Geometry check sheet. Reference: the model listing, model coordinates, mm. A direction names the side the tool comes from. Coordinates: 2 decimals unless noted, no trailing zeros. Write each loop counter-clockwise with the first axis right and the second up, starting at its lowest first coordinate (ties: lowest second). Pieces come first, ordered by that corner, then holes. Notation, with made-up numbers: M -34.5,60.5 L -21.5,60.5 A37 ccw -21.5,98.5 Z; hole C 79,-21 d9. An arc over 180 degrees is marked long. Write item = value, one per line. Start each with the question number.
```python
from build123d import *

# Parameters (mm, degrees)
SKETCH1_R           = 1.5
BOSS_EXTRUDE1_DEPTH = 1
SKETCH2_W           = 15.22
SKETCH2_H           = 11.45
BOSS_EXTRUDE2_DEPTH = 5.3
SKETCH3_W           = 13.43
SKETCH3_H           = 1.95
BOSS_EXTRUDE3_DEPTH = 3.5
SKETCH5_W           = 7.6
SKETCH5_H           = 3.8
BOSS_EXTRUDE4_DEPTH = 1.65
SKETCH4_W           = 13.22
SKETCH4_H           = 3.3
SKETCH4_W_2         = 5.6
SKETCH4_H_2         = 1.65
SKETCH4_W_3         = 1.3
SKETCH4_H_3         = 1
CUT_EXTRUDE1_DEPTH  = 9.3
SKETCH6_W           = 0.8
SKETCH6_H           = 0.8
BOSS_EXTRUDE5_DEPTH = 5.95
SKETCH7_W           = 4
SKETCH7_H           = 5.1
BOSS_EXTRUDE6_DEPTH = 1.6
FILLET1_R           = 0.25


with BuildPart() as part:
    # Sketch1 → Boss-Extrude1 (new body)
    with BuildSketch(Plane(origin=(0, 0, 0), x_dir=(1, 0, 0), z_dir=(0, 1, 0))):
        with BuildLine():
            ThreePointArc((-11.9, -8.825), (-10.999353352, -10.999353352), (-8.825, -11.9))
            Line((-8.825, -11.9), (8.825, -11.9))
            ThreePointArc((8.825, -11.9), (10.999353352, -10.999353352), (11.9, -8.825))
            Line((11.9, -8.825), (11.9, 8.825))
            ThreePointArc((11.9, 8.825), (10.999353357, 10.999353347), (8.825000015, 11.9))
            Line((8.825000015, 11.9), (-8.825, 11.9))
            ThreePointArc((-8.825, 11.9), (-10.999353347, 10.999353357), (-11.9, 8.825000015))
            Line((-11.9, 8.825000015), (-11.9, -8.825))
        make_face()
        with Locations((8.825, -8.825)):
            Circle(SKETCH1_R, mode=Mode.SUBTRACT)
        with Locations((-8.825, -8.825)):
            Circle(SKETCH1_R, mode=Mode.SUBTRACT)
        with Locations((-8.825, 8.825)):
            Circle(SKETCH1_R, mode=Mode.SUBTRACT)
        with Locations((8.825, 8.825)):
            Circle(SKETCH1_R, mode=Mode.SUBTRACT)
    extrude(amount=BOSS_EXTRUDE1_DEPTH)

    # Sketch2 → Boss-Extrude2 (add)
    with BuildSketch(Plane(origin=(0, 1, 0), x_dir=(1, 0, 0), z_dir=(0, 1, 0))):
        Rectangle(SKETCH2_W, SKETCH2_H)
    extrude(amount=BOSS_EXTRUDE2_DEPTH)

    # Sketch3 → Boss-Extrude3 (add)
    with BuildSketch(Plane(origin=(0, 1, 0), x_dir=(1, 0, 0), z_dir=(0, 1, 0))):
        with Locations((0, 6.7)):
            Rectangle(SKETCH3_W, SKETCH3_H)
    extrude(amount=BOSS_EXTRUDE3_DEPTH)

    # Sketch5 → Boss-Extrude4 (add)
    with BuildSketch(Plane(origin=(0, 6.3, 0), x_dir=(1, 0, 0), z_dir=(0, 1, 0))):
        with Locations((0, -3.825)):
            Rectangle(SKETCH5_W, SKETCH5_H)
    extrude(amount=BOSS_EXTRUDE4_DEPTH)

    # Sketch4 → Cut-Extrude1 (cut)
    with BuildSketch(Plane.XY.offset(5.725)):
        with Locations((0, 3.65)):
            Rectangle(SKETCH4_W, SKETCH4_H)
        with Locations((0, 6.125)):
            Rectangle(SKETCH4_W_2, SKETCH4_H_2)
        with Locations((-3.76, 1.5)):
            Rectangle(SKETCH4_W_3, SKETCH4_H_3)
        with Locations((3.76, 1.5)):
            Rectangle(SKETCH4_W_3, SKETCH4_H_3)
    extrude(amount=-CUT_EXTRUDE1_DEPTH, mode=Mode.SUBTRACT)

    # Sketch6 → Boss-Extrude5 (add)
    with BuildSketch(Plane.XY.offset(-3.575)):
        with Locations((2.54, 3.65)):
            Rectangle(SKETCH6_W, SKETCH6_H)
        with Locations((0, 3.65)):
            Rectangle(SKETCH6_W, SKETCH6_H)
        with Locations((5.08, 3.65)):
            Rectangle(SKETCH6_W, SKETCH6_H)
        with Locations((-2.54, 3.65)):
            Rectangle(SKETCH6_W, SKETCH6_H)
        with Locations((-5.08, 3.65)):
            Rectangle(SKETCH6_W, SKETCH6_H)
    extrude(amount=BOSS_EXTRUDE5_DEPTH)

    # Sketch7 → Boss-Extrude6 (add)
    with BuildSketch(Plane.XZ):
        Rectangle(SKETCH7_W, SKETCH7_H)
    extrude(amount=BOSS_EXTRUDE6_DEPTH)

    # Fillet1
    fillet1_edges = [part.edges().sort_by_distance(p)[0] for p in [
        (2, -1.6, 0),
        (0, -1.6, 2.55),
        (-2, -1.6, 0),
        (0, -1.6, -2.55),
    ]]
    fillet(fillet1_edges, radius=FILLET1_R)


solid = part.part
```
Q1. Gauge pin test, flat ends, axial feed: pin 1 (1 mm diameter, centred on y = 6.5, z = 6, fed in from +X); pin 2 (1.5 mm diameter, centred on y = 6.5, z = 8, fed in from +X) (3 decimals); pin 3 (2 mm diameter, centred on x = 6, y = 4.5, fed in from +Z) (3 decimals); pin 4 (1.6 mm diameter, centred on x = 2.5, y = 5, fed in from -Z) (3 decimals). Record the tip position at first contact, or that the pin passes through.
Q2. Draft check along X on faces 6 (the face through (0, 7.95, 4)), 7 (the face through (-3.8, 7, 4)), 8 (the face through (4.41, 1.5, 1.1)), 9 (the face through (7.61, 4, 0)). Enter one of: pulls with the +X half, pulls with the -X half, needs draft (parallel to the pull), parting line crosses it, or undercut.
Q3. Set-up check for faces 1 (the face through (-7.61, 4, 0)), 2 (the face through (0, 7.3, 5.725)), 3 (the face through (11.9, 0.5, 0.1)), 4 (the face through (7.635, 0.493, 9.738)), 5 (the face through (-5, 4.05, -1)): record each of +Z, -Z, +X, -X, +Y, -Y from which the full face is reachable in a straight line by a thin tool's end or side.
Q4. Cross-section at D-D on x = 6. Enter the section's corners in (y, z) (3 decimals).
Q5. Cross-section at B-B on y = 2.5. Enter the section's corners in (x, z) (3 decimals).
Q6. Cross-section at A-A on x = 1.25. Enter the section's corners in (y, z) (3 decimals).
Q7. Scan lines: L1, parallel to X at y = 1.25, z = 4.25; L2, parallel to Y at x = -4.25, z = -3.5; L3, parallel to X at y = 5.5, z = 1.75. Record each from-to range of solid material in increasing order.
Q8. Cross-section at C-C on z = 9.75. Enter the section's corners in (x, y), and give its area (3 significant figures).
Values found:
q1.pin_1 = 7.61
q1.pin_2 = through
q1.pin_3 = 5.725
q1.pin_4 = -7.675
q2.face_6 = needs draft
q2.face_7 = pulls with the -X half
q2.face_8 = undercut
q2.face_9 = pulls with the +X half
q3.face_1 = +Z, -Z, -X, +Y
q3.face_2 = +Z, +X, -X, +Y
q3.face_3 = +Z, -Z, +X, +Y, -Y
q3.face_4 = +Y, -Y
q3.face_5 = +Z
q4.outline = M 0,-11.9 L 1,-11.9 L 1,-7.675 L 4.5,-7.675 L 4.5,-5.725 L 6.3,-5.725 L 6.3,5.725 L 5.3,5.725 L 5.3,-3.575 L 2,-3.575 L 2,5.725 L 1,5.725 L 1,11.9 L 0,11.9 Z
q5.outline = M -7.61,-5.725 L -6.715,-5.725 L -6.715,-7.675 L 6.715,-7.675 L 6.715,-5.725 L 7.61,-5.725 L 7.61,5.725 L 6.61,5.725 L 6.61,-3.575 L -6.61,-3.575 L -6.61,5.725 L -7.61,5.725 Z
q6.outline = M -1.6,-2.3 A0.25 ccw -1.35,-2.55 L 0,-2.55 L 0,-11.9 L 1,-11.9 L 1,-7.675 L 4.5,-7.675 L 4.5,-5.725 L 6.3,-5.725 L 6.3,-3.575 L 2,-3.575 L 2,5.725 L 1,5.725 L 1,11.9 L 0,11.9 L 0,2.55 L -1.35,2.55 A0.25 ccw -1.6,2.3 Z; M 6.95,1.925 L 7.95,1.925 L 7.95,5.725 L 6.95,5.725 Z
q7.L1 = -7.61 to -4.41, -3.11 to 3.11, 4.41 to 7.61
q7.L2 = 0 to 1, 5.3 to 6.3
q7.L3 = -7.61 to -2.8, 2.8 to 7.61
q8.outline = M -11.76,0 L -10.01,0 L -10.01,1 L -11.76,1 Z; M -7.64,0 L 7.64,0 L 7.64,1 L -7.64,1 Z; M 10.01,0 L 11.76,0 L 11.76,1 L 10.01,1 Z
q8.area = 18.8 mm²
